Work out the finished part from the listing and answer in its coordinate system (mm). Face numbers are marked on the shaded views. Round coordinates to 2 decimals unless told otherwise and drop trailing zeros. Loops run counter-clockwise (first coordinate to the right, second up) from the corner with the lowest first, then second, coordinate; pieces in that order, holes last. Notation, with made-up numbers: (0.5, 28.25) -> (11.5, 28.25) arc R21 ccw to (11.5, 58.25) -> close; hole circle Ø10 at (56.5, -40). An arc over 180 degrees is marked (long way). Use CSV: the item, a comma, the result in double quotes. Start each with the question number.
from build123d import *

# Parameters (mm, degrees)
F0_W     = 13.97
F0_H     = 40.005
F1_DEPTH = 3.175
F2_DEPTH = 2.54
F5_DEPTH = 25.4
F6_DEPTH = 3.81
F7_R     = 0.2286
F8_R     = 0.2286
F9_R     = 0.254


with BuildPart() as f1:
    # F0 (on Front) → F1 (new body)
    with BuildSketch(Plane.XZ):
        Rectangle(F0_W, F0_H)
    extrude(amount=F1_DEPTH)

    # F2 (cut): a face of the model
    f2_faces = [f1.faces().sort_by_distance(p)[0] for p in [
        (0, 0, 0),
    ]]
    extrude(f2_faces, amount=-F2_DEPTH, mode=Mode.SUBTRACT)

    # F3 (on face) → F5 (cut)
    with BuildSketch(Plane.XZ.offset(3.175)):
        with BuildLine():
            Line((2.6061468011, 4.583747707), (2.6061468011, 13.593294405))
            ThreePointArc((2.6061468011, 13.593294405), (1.8441656406, 15.4357593505), (0.003389831, 16.201812079))
            ThreePointArc((0.003389831, 16.201812079), (0.001844595, 16.2018134827), (0.0002993585, 16.2018139709))
            Line((0.0002993585, 16.2018139709), (0.0002993585, 1.9778139709))
            ThreePointArc((0.0002993585, 1.9778139709), (0.9737013076, 2.1662350173), (1.8064818654, 2.704278127))
            ThreePointArc((1.8064818654, 2.704278127), (2.3979195865, 3.5624899149), (2.6061468011, 4.583747707))
        make_face()
        with BuildLine():
            Line((0.0002993585, 1.9778139709), (0.0002993585, 16.2018139709))
            ThreePointArc((0.0002993585, 16.2018139709), (-1.8401435929, 15.4418995197), (-2.6082506073, 13.6048606402))
            Line((-2.6082506073, 13.6048606402), (-2.6082570215, 4.5863722062))
            ThreePointArc((-2.6082570215, 4.5863722062), (-1.8442292029, 2.7418431015), (0.0002993585, 1.9778139709))
        make_face()
    extrude(amount=-F5_DEPTH, mode=Mode.SUBTRACT)

    # F4 (on face) → F6 (join)
    with BuildSketch(Plane.XZ.offset(3.175)):
        Polygon((-5.783022847, 2.1209), (-4.513022847, 2.1209), (-4.513022847, 17.5387), (4.5277241152, 17.5387), (4.5277241152, 2.1209), (5.7977241152, 2.1209), (5.7977241152, 18.8087), (-5.783022847, 18.8087), align=None)
    extrude(amount=F6_DEPTH)

    # F7
    f7_edges = [f1.edges().sort_by_distance(p)[0] for p in [
        (6.985, -2.54, 0),
        (0, -2.54, -20.0025),
        (0, -2.54, 20.0025),
        (-6.985, -2.54, 0),
        (2.39792, -2.54, 3.56249),
        (2.606147, -2.54, 9.088521),
        (1.844166, -2.54, 15.435759),
        (0.001845, -2.54, 16.201813),
        (-1.840144, -2.54, 15.4419),
        (-2.608254, -2.54, 9.095616),
        (-1.022696, -2.54, 2.186777),
    ]]
    fillet(f7_edges, radius=F7_R)

    # F8
    f8_edges = [f1.edges().sort_by_distance(p)[0] for p in [
        (6.985, -3.175, 0),
        (0, -3.175, -20.0025),
        (0, -3.175, 20.0025),
        (-6.985, -3.175, 0),
        (2.39792, -3.175, 3.56249),
        (-1.022696, -3.175, 2.186777),
        (2.606147, -3.175, 9.088521),
        (-2.608254, -3.175, 9.095616),
        (1.844166, -3.175, 15.435759),
        (-1.840144, -3.175, 15.4419),
        (0.001845, -3.175, 16.201813),
        (-5.148023, -3.175, 2.1209),
        (-4.513023, -3.175, 9.8298),
        (0.007351, -3.175, 17.5387),
        (4.527724, -3.175, 9.8298),
        (5.162724, -3.175, 2.1209),
        (5.797724, -3.175, 10.4648),
        (0.007351, -3.175, 18.8087),
        (-5.783023, -3.175, 10.4648),
    ]]
    fillet(f8_edges, radius=F8_R)

    # F9
    f9_edges = [f1.edges().sort_by_distance(p)[0] for p in [
        (-5.148023, -6.985, 2.1209),
        (-4.513023, -6.985, 9.8298),
        (0.007351, -6.985, 17.5387),
        (4.527724, -6.985, 9.8298),
        (5.162724, -6.985, 2.1209),
        (5.797724, -6.985, 10.4648),
        (0.007351, -6.985, 18.8087),
        (-5.783023, -6.985, 10.4648),
    ]]
    fillet(f9_edges, radius=F9_R)


solid = f1.part
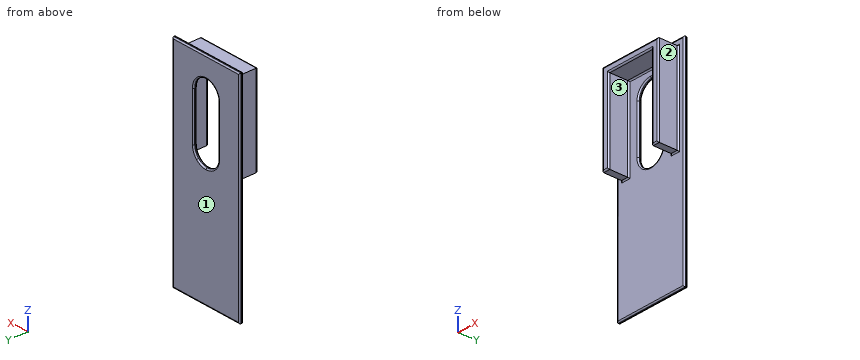
Q1. Section C-C, the plane z = -14.5 is taken. Write down the section's boundary in (x, y) (3 decimals), and give its area (3 significant figures).
Q2. Each of these flat-tipped pins is pushed along its axis until it touches: pin 1 (1 mm diameter, centred on x = -4.5, y = -5.5, fed in from +Z); pin 2 (1.7 mm diameter, centred on y = -5, z = 7, fed in from +X); pin 3 (2 mm diameter, centred on y = -5, z = 13.5, fed in from -X). Where does it stop, or does it pass through?
Q3. Straight lines are drawn through the part: line 1 (X direction, y = -3, z = 7.5); line 2 (X direction, y = -4.25, z = 13); line 3 (Z direction, x = -3.5, y = -5.75). For each, find the intervals that lie inside material, in ascending order. Write a range as from..to.
Q4. Section B-B, the plane y = -5.5 is taken. Write down the section's boundary in (x, z), and give its area (3 significant figures).
Q5. For a pull along X with two mould halves and no side action, classify the marked faces 1, 2 and 3 as pulls with the +X half, pulls with the -X half, needs draft (parallel to the pull), parting line crosses it, or undercut.
Report:
1,outline,"(-6.985, -2.946) arc R0.229 ccw to (-6.756, -3.175) -> (6.756, -3.175) arc R0.229 ccw to (6.985, -2.946) -> (6.985, -2.769) arc R0.229 ccw to (6.756, -2.54) -> (-6.756, -2.54) arc R0.229 ccw to (-6.985, -2.769) -> close"
1,area,"8.83 mm²"
2,pin 1,"stops at z = 18.81"
2,pin 2,"stops at x = 5.8"
2,pin 3,"stops at x = -5.78"
3,line 1,"x = -6.98..-2.61, 2.61..6.98"
3,line 2,"x = -5.78..-4.51, 4.53..5.8"
3,line 3,"z = 17.54..18.81"
4,outline,"(-5.78, 2.12) -> (-4.51, 2.12) -> (-4.51, 17.54) -> (4.53, 17.54) -> (4.53, 2.12) -> (5.8, 2.12) -> (5.8, 18.81) -> (-5.78, 18.81) -> close"
4,area,"53.9 mm²"
5,face 1,"needs draft"
5,face 2,"pulls with the +X half"
5,face 3,"undercut"
